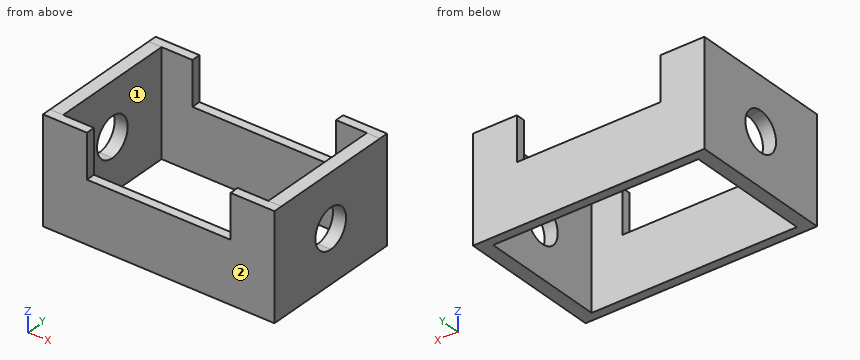
from build123d import *
from build123d import SkipClean  # not in build123d's __all__

# Parameters (mm, degrees)
F0_W     = 4.6070814133
F0_H     = 36.8574000895
F1_DEPTH = 3.175
F2_DEPTH = 25.4
F4_DEPTH = 6.35


# Not quite as in the source:
# - a feature names something its author has since deleted; it is built from what else it names


with BuildPart() as f1:
    # F0 (on Front) → F1 (new body)
    with BuildSketch(Plane.XZ):
        with Locations((38.3936055005, 18.4287000448)):
            Rectangle(F0_W, F0_H)
        Polygon((0, 21.4239992201), (0, 0), (36.0900647938, 0), (36.0900647938, 36.8574000895), (25.2613946795, 36.8574000895), (25.2613946795, 21.4239992201), align=None)
        Polygon((0, 21.4239992201), (0, 0), (36.0900647938, 0), (36.0900647938, 36.8574000895), (25.2613946795, 36.8574000895), (25.2613946795, 21.4239992201), align=None)
    extrude(amount=F1_DEPTH)

    # F0 (on Front) → F2 (join)
    with BuildSketch(Plane.XZ):
        with Locations((38.3936055005, 18.4287000448)):
            Rectangle(F0_W, F0_H)
    extrude(amount=F2_DEPTH)

    # F3 (on face) → F4 (cut)
    with BuildSketch(Plane.YZ.offset(40.6971462071)):
        with BuildLine():
            Line((-25.4, 25.344834663), (-25.4, 11.5125654265))
            ThreePointArc((-25.4, 11.5125654265), (-18.4838653818, 18.4287000448), (-25.4, 25.344834663))
        make_face()
    extrude(amount=-F4_DEPTH, mode=Mode.SUBTRACT)

    # F5: F1 across plane


with BuildPart() as f1_1:
    add(f1.part, clean=False)
    add(f1.part.mirror(Plane.YZ), clean=False)

    # F6: F1 across face


with BuildPart() as f1_2:
    add(f1_1.part, clean=False)
    with SkipClean():  # cleaning this boolean's faces spoils the solid; the shape is the same uncleaned
        add(f1_1.part.mirror(Plane(origin=(38.3936055005, -25.4, 5.7562827133), x_dir=(1, 0, 0), z_dir=(0, -1, 0))), clean=False)


solid = f1_2.part
Could you check a few things on this model? Use its own coordinates, in mm. Face numbers are marked on the shaded views. A direction names the side the tool comes from. Give positions to 0.01 mm unless a question says otherwise; leave off trailing zeros. Order: outer loops, then holes, each group sorted by start corner. A loop starts at its lowest first (then second) coordinate and runs counter-clockwise, first axis right, second up. Notation, with made-up numbers: (-20, 52.25) - (-11, 52.25) arc R17 ccw to (-11, 82.25) - close; hole circle Ø5 at (-25, -19.5). An arc over 180 degrees is marked (long way). One line per item, written item: value. Start each with the question number.
1. For the marked faces 1 and 2, which set-ups out of +Z, -Z, +X, -X, +Y, -Y let a thin tool reach every point of the face, with its end or its side?
2. For P1, Ø1.6, axis at x = 11, y = -1, coming from the +Z side, with a flat end and sliding along its axis, tell me the tip position at first contact or that it passes through.
3. Imagine slicing it at B-B on x = 2. List the corners of the cut face in (y, z) for me (3 decimals).
4. If I drill on probe 1 along X at (y, z) = (-40.5, 35.5); probe 2 along Y at (x, z) = (15, 10.5) (3 decimals); probe 3 along Z at (x, y) = (14, -48), over which ranges is the centre line in solid material (lowest first)?
5. Imagine slicing it at C-C on z = 10. List the corners of the cut face in (x, y) for me (3 decimals).
6. Imagine slicing it at A-A on y = -11. List the corners of the cut face in (x, z) for me, plus the area to 3 significant figures.
Values:
1. face 1: +Z, -Z
1. face 2: +Z, -Z, +X, -X, -Y
2. P1: z = 21.42
3. outline: (-50.8, 0) - (-47.625, 0) - (-47.625, 21.424) - (-50.8, 21.424) - close; (-3.175, 0) - (0, 0) - (0, 21.424) - (-3.175, 21.424) - close
4. probe 1: -40.7 to -36.09, 36.09 to 40.7
4. probe 2: -50.8 to -47.625, -3.175 to 0
4. probe 3: 0 to 21.42
5. outline: (-40.697, -50.8) - (40.697, -50.8) - (40.697, 0) - (-40.697, 0) - close; hole (-36.09, -47.625) - (36.09, -47.625) - (36.09, -3.175) - (-36.09, -3.175) - close
6. outline: (-40.7, 0) - (-36.09, 0) - (-36.09, 36.86) - (-40.7, 36.86) - close; (36.09, 0) - (40.7, 0) - (40.7, 36.86) - (36.09, 36.86) - close
6. area: 340 mm²
